Work out the finished part from the listing and answer in its coordinate system (mm). A direction names the side the tool comes from. Coordinates: 2 decimals unless noted, no trailing zeros. Write each question's results on one line, items separated by ' | '. Start each with the question number.
Item 1: Section A-A, the plane x = 5 is taken. Count the separate pieces of the cut face and the enclosed holes in it, plus the area to 3 significant figures.
Item 2: For a pull along Y with two mould halves and no side action, classify faces 1 (the face through (9, 114.3, -437)), 2 (the face through (9, 63.5, -853)), 3 (the face through (9, 0, -425)) as +Y half, -Y half, draft (parallel to the pull), parting line (faces both ways), or undercut.
Item 3: A tool of negligible diameter and unlimited length cuts with its end or side. For faces 4 (the face through (19.05, 58, -425)), 5 (the face through (9, 101.6, -853)), 6 (the face through (9, 76.2, -9)), from which of +Z, -Z, +X, -X, +Y, -Y can it reach the whole face along a straight path? Write none if from no direction.
Item 4: Consider probe 1 along Z at (x, y) = (16.5, 97); probe 2 along Z at (x, y) = (5.5, 17.5); probe 3 along Z at (x, y) = (11.5, 93.5). Determine where each line is inside the solid, lowest interval first. Write a range as [from, to].
Item 5: Each of these flat-tipped pins is pushed along its axis until it touches: pin 1 Ø6.5 at (y, z) = (95.25, -49.06) entering from +X; pin 2 Ø6.5 at (x, y) = (8.5, 43.5) entering from +Z; pin 3 Ø8 at (x, y) = (12.5, 68.5) entering from -Z. Where does it stop, or does it pass through?
from build123d import *

# Parameters (mm, degrees)
BOSS_EXTRUDE1_DEPTH             = 19.05
F_7_32_0_21875_DIAMETER_HOLE2_D = 5.55625


with BuildPart() as part:
    # Sketch1 → Boss-Extrude1 (new body)
    with BuildSketch(Plane(origin=(0, 0, 0), x_dir=(0, 0, -1), z_dir=(1, 0, 0))):
        Polygon((0, 0), (862.33, 0), (862.33, 12.7), (843.28, 12.7), (843.28, 25.4), (862.33, 25.4), (862.33, 38.1), (843.28, 38.1), (843.28, 50.8), (862.33, 50.8), (862.33, 63.5), (843.28, 63.5), (843.28, 76.2), (862.33, 76.2), (862.33, 88.9), (843.28, 88.9), (843.28, 101.6), (862.33, 101.6), (862.33, 114.3), (0, 114.3), (0, 101.6), (19.05, 101.6), (19.05, 88.9), (0, 88.9), (0, 76.2), (19.05, 76.2), (19.05, 63.5), (0, 63.5), (0, 50.8), (19.05, 50.8), (19.05, 38.1), (0, 38.1), (0, 25.4), (19.05, 25.4), (19.05, 12.7), (0, 12.7), align=None)
    extrude(amount=BOSS_EXTRUDE1_DEPTH)

    # 7/32 (0.21875) Diameter Hole2 (through all)
    with Locations(Plane(origin=(19.05, 0, 0), x_dir=(0, 0, -1), z_dir=(1, 0, 0))):
        with Locations((49.0601, 55.499), (99.8601, 55.499), (232.38206, 55.499), (364.90402, 55.499), (497.42598, 55.499), (629.94794, 55.499), (762.4699, 55.499), (813.2699, 55.499), (813.2699, 95.25), (813.2699, 19.05), (49.0601, 95.25), (49.0601, 19.05), (90.968322508, 93.8784), (107.478322508, 93.8784)):
            Hole(F_7_32_0_21875_DIAMETER_HOLE2_D / 2)


solid = part.part
Answer key:
1) separate pieces: 1 | enclosed holes: 14 | area: 96,300 mm^2
2) face 1: +Y half | face 2: undercut | face 3: -Y half
3) face 4: +Z, -Z, +X, +Y, -Y | face 5: -Z, +X, -X | face 6: +Z, +X, -X
4) probe 1: z = [-843.28, -815.43], [-811.11, -51.22], [-46.9, -19.05] | probe 2: z = [-843.28, -815.58], [-810.96, -51.37], [-46.75, -19.05] | probe 3: z = [-843.28, -815.43], [-811.11, -110.23], [-104.73, -93.72], [-88.22, -51.22], [-46.9, -19.05]
5) pin 1: stops at x = 19.05 | pin 2: stops at z = -19.05 | pin 3: stops at z = -843.28
